Source: CAD feature listing. Evaluate the final solid. Frame: model axes, mm. A direction names the side the tool comes from. Round coordinates to 2 decimals unless told otherwise and drop trailing zeros. Loops run counter-clockwise (first coordinate to the right, second up) from the corner with the lowest first, then second, coordinate; pieces in that order, holes last. Notation, with made-up numbers: M 23,12.5 L 44,12.5 A15 ccw 44,33.5 Z; hole C 54,16 d9. An arc over 180 degrees is marked long. One line per item, written item: value.
from build123d import *

# Parameters (mm, degrees)
SKETCH_1_R               = 25.75
SKETCH_1_R_2             = 24
EXTRUDE_1_DEPTH          = 30
SKETCH_2_R               = 37
SKETCH_2_R_2             = 24
EXTRUDE_2_DEPTH          = 3
SKETCH_3_R               = 29
CUT_EXTRUDE_1_DEPTH      = 1
SKETCH_4_R               = 1.6
CUT_EXTRUDE_2_DEPTH      = 21
PATTERN_CIRCULAR_1_COUNT = 6
SKETCH_5_R               = 22
CUT_EXTRUDE_3_DEPTH      = 11
PATTERN_CIRCULAR_2_COUNT = 6
SKETCH_6_R               = 25.75
SKETCH_6_R_2             = 10
EXTRUDE_3_DEPTH          = 2
SKETCH_7_R               = 12
SKETCH_7_R_2             = 10
EXTRUDE_4_DEPTH          = 13
SKETCH_8_R               = 4
CUT_EXTRUDE_5_DEPTH      = 15.3
PATTERN_CIRCULAR_4_COUNT = 4
SKETCH_9_R               = 10
SKETCH_9_R_2             = 9
EXTRUDE_5_DEPTH          = 2
FILLET_1_R               = 10


with BuildPart() as part:
    # 草图1 → 凸台-拉伸1 (new body)
    with BuildSketch(Plane(origin=(0, 0, 0), x_dir=(1, 0, 0), z_dir=(0, 1, 0))):
        with Locations(Location((0, 0, 0), (0, 0, 270))):
            Circle(SKETCH_1_R)
        with Locations(Location((0, 0, 0), (0, 0, 270))):
            Circle(SKETCH_1_R_2, mode=Mode.SUBTRACT)
    extrude(amount=EXTRUDE_1_DEPTH)

    # 草图2 → 凸台-拉伸2 (add)
    with BuildSketch(Plane.XZ):
        with Locations(Location((0, 0, 0), (0, 0, 270))):
            Circle(SKETCH_2_R)
        with Locations(Location((0, 0, 0), (0, 0, 90))):
            Circle(SKETCH_2_R_2, mode=Mode.SUBTRACT)
    extrude(amount=-EXTRUDE_2_DEPTH)

    # 草图3 → 切除-拉伸1 (cut)
    with BuildSketch(Plane.XZ):
        with Locations(Location((0, 0, 0), (0, 0, 270))):
            Circle(SKETCH_3_R)
    extrude(amount=-CUT_EXTRUDE_1_DEPTH, mode=Mode.SUBTRACT)

    # 草图4 → 切除-拉伸2 (cut)
    with BuildSketch(Plane(origin=(0, 3, 0), x_dir=(1, 0, 0), z_dir=(0, 1, 0))):
        with Locations(Location((0, 33.5, 0), (0, 0, 270))):
            Circle(SKETCH_4_R)
    cut_extrude_2 = extrude(amount=-CUT_EXTRUDE_2_DEPTH, mode=Mode.SUBTRACT)

    # 阵列(圆周)1: 切除-拉伸2 ×6 about axis
    pattern_circular_1_axis = Axis((0, 0, 0), (0, 1, 0))
    for i in range(1, PATTERN_CIRCULAR_1_COUNT):
        add(cut_extrude_2.rotate(pattern_circular_1_axis, i * 360 / PATTERN_CIRCULAR_1_COUNT), mode=Mode.SUBTRACT)

    # 草图5 → 切除-拉伸3 (cut)
    with BuildSketch(Plane.XZ):
        with Locations((56, 0)):
            Circle(SKETCH_5_R)
    cut_extrude_3 = extrude(amount=-CUT_EXTRUDE_3_DEPTH, mode=Mode.SUBTRACT)

    # 阵列(圆周)2: 切除-拉伸3 ×6 about axis
    pattern_circular_2_axis = Axis((0, 0, 0), (0, 1, 0))
    for i in range(1, PATTERN_CIRCULAR_2_COUNT):
        add(cut_extrude_3.rotate(pattern_circular_2_axis, i * 360 / PATTERN_CIRCULAR_2_COUNT), mode=Mode.SUBTRACT)

    # 草图6 → 凸台-拉伸3 (add)
    with BuildSketch(Plane(origin=(0, 30, 0), x_dir=(1, 0, 0), z_dir=(0, 1, 0))):
        with Locations(Location((0, 0, 0), (0, 0, 90))):
            Circle(SKETCH_6_R)
        with Locations(Location((0, 0, 0), (0, 0, 270))):
            Circle(SKETCH_6_R_2, mode=Mode.SUBTRACT)
    extrude(amount=EXTRUDE_3_DEPTH)

    # 草图7 → 凸台-拉伸4 (add)
    with BuildSketch(Plane(origin=(0, 32, 0), x_dir=(1, 0, 0), z_dir=(0, 1, 0))):
        with Locations(Location((0, 0, 0), (0, 0, 90))):
            Circle(SKETCH_7_R)
        with Locations(Location((0, 0, 0), (0, 0, 270))):
            Circle(SKETCH_7_R_2, mode=Mode.SUBTRACT)
    extrude(amount=EXTRUDE_4_DEPTH)

    # 草图8 → 切除-拉伸5 (cut)
    with BuildSketch(Plane(origin=(0, 32, 0), x_dir=(1, 0, 0), z_dir=(0, 1, 0))):
        with Locations(Location((0, 17.5, 0), (0, 0, 270))):
            Circle(SKETCH_8_R)
    cut_extrude_5 = extrude(amount=-CUT_EXTRUDE_5_DEPTH, mode=Mode.SUBTRACT)

    # 阵列(圆周)4: 切除-拉伸5 ×4 about axis
    pattern_circular_4_axis = Axis((0, 0, 0), (0, 1, 0))
    for i in range(1, PATTERN_CIRCULAR_4_COUNT):
        add(cut_extrude_5.rotate(pattern_circular_4_axis, i * 360 / PATTERN_CIRCULAR_4_COUNT), mode=Mode.SUBTRACT)

    # 草图9 → 凸台-拉伸5 (add)
    with BuildSketch(Plane.XZ.offset(-30)):
        with Locations(Location((0, 0, 0), (0, 0, 270))):
            Circle(SKETCH_9_R)
        with Locations(Location((0, 0, 0), (0, 0, 270))):
            Circle(SKETCH_9_R_2, mode=Mode.SUBTRACT)
    extrude(amount=-EXTRUDE_5_DEPTH)

    # 圆角1
    fillet_1_edges = [part.edges().sort_by_distance(p)[0] for p in [
        (35.901785714, 1.5, -8.947724992),
        (35.901785714, 1.5, 8.947724992),
        (25.699850006, 1.5, 26.617995974),
        (10.201935708, 1.5, 35.565720966),
        (-10.201935708, 1.5, 35.565720966),
        (-25.699850006, 1.5, 26.617995974),
        (-35.901785714, 1.5, 8.947724992),
        (-35.901785714, 1.5, -8.947724992),
        (-25.699850006, 1.5, -26.617995974),
        (-10.201935708, 1.5, -35.565720966),
        (10.201935708, 1.5, -35.565720966),
        (25.699850006, 1.5, -26.617995974),
    ]]
    fillet(fillet_1_edges, radius=FILLET_1_R)


solid = part.part
1. Section query D-D (x = -15). Return the cut outline in (y, z) (1 decimal).
Report:
outline: M 0,-30.7 L 3,-30.7 L 3,-20.9 L 32,-20.9 L 32,-3.1 L 30,-3.1 L 30,-18.7 L 1,-18.7 L 1,-24.8 L 0,-24.8 Z; M 0,24.8 L 1,24.8 L 1,18.7 L 30,18.7 L 30,3.1 L 32,3.1 L 32,20.9 L 3,20.9 L 3,30.7 L 0,30.7 Z
2. Section query B-B (x = 0). Count the separate pieces of the cut face and the enclosed holes in it, and give its area (3 significant figures).
Report:
separate pieces: 6
enclosed holes: 0
area: 230 mm2
3. Pin query (flat end, axial travel): pin 1 (17.5 mm diameter, centred on x = -11.5, z = 9, fed in from -Y); pin 2 (3.5 mm diameter, centred on x = -29.01, z = 16.75, fed in from +Y); pin 3 (8 mm diameter, centred on x = 10.5, z = 24.5, fed in from +Y). Return the tip coordinate at first contact, or that it passes through.
Report:
pin 1: stops at y = 30
pin 2: stops at y = 3
pin 3: stops at y = 32
4. Section query C-C (y = 29). Return the cut outline in (x, z).
Report:
outline: C 0,0 d51.5; hole C 0,0 d48
5. Section query A-A (x = 17.5). Return the cut outline in (y, z).
Report:
outline: M 0,-29.16 L 3,-29.16 L 3,-18.89 L 32,-18.89 L 32,-4 L 30,-4 L 30,-16.42 L 1,-16.42 L 1,-23.12 L 0,-23.12 Z; M 0,23.12 L 1,23.12 L 1,16.42 L 30,16.42 L 30,4 L 32,4 L 32,18.89 L 3,18.89 L 3,29.16 L 0,29.16 Z
6. Reachability of faces 1 (the face through (0, 30, -10)), 2 (the face through (5.4, 32, -11.1)), 3 (the face through (27.425, 1.521, -16.542)) from +Z, -Z, +X, -X, +Y, -Y: full face, straight path, thin tool, end or side. Return the list, or none.
Report:
face 1: -Y
face 2: +Y
face 3: +Y, -Y
7. Ray query, line 1 (Z direction, x = -0.5, y = 4.5); line 2 (Y direction, x = 19.5, z = -18); line 3 (X direction, y = 21, z = 0). Return the intervals inside material, ascending. Write a range as [from, to].
Report:
line 1: z = [-25.75, -23.99], [23.99, 25.75]
line 2: y = [1, 3]
line 3: x = [-25.75, -24], [24, 25.75]
8. Pull-direction query (X, two-part tool) for faces 4 (the face through (2.703, 30.986, -8.584)), 5 (the face through (-17.08, 1.48, 29.4)), 6 (the face through (32.1, 1.5, 18.4)), 7 (the face through (-9, 45, 5)); classes: released by +X, released by -X, zero draft, split by the parting line, or undercut.
Report:
face 4: undercut
face 5: released by -X
face 6: released by +X
face 7: zero draft
